Input: part model. Units: mm. Frame: model coordinates. A direction names the side the tool comes from. Give positions to 0.01 mm unless a question says otherwise; leave off trailing zeros. Order: outer loops, then holes, each group sorted by start corner. A loop starts at its lowest first (then second) coordinate and runs counter-clockwise, first axis right, second up.
```python
from build123d import *

# Parameters (mm, degrees)
F0_W           = 50
F0_H           = 45
F1_DEPTH       = 30
F2_SIZE        = 10
F4_D           = 8.8
F4_CBORE_D     = 14.25
F4_CBORE_DEPTH = 8
F5_DEPTH       = 50


with BuildPart() as f1:
    # F0 (on Top) → F1 (new body)
    with BuildSketch(Plane.XY):
        with Locations((-2.2690217942, 1.8614111841)):
            Rectangle(F0_W, F0_H)
    extrude(amount=F1_DEPTH)

    # F2
    f2_edges = [f1.edges().sort_by_distance(p)[0] for p in [
        (-27.269022, 24.361411, 15),
        (22.730978, -20.638589, 15),
        (22.730978, 24.361411, 15),
        (-27.269022, -20.638589, 15),
    ]]
    chamfer(f2_edges, length=F2_SIZE)

    # F4 (through all)
    with Locations(Plane.XY.offset(30)):
        with Locations((-17.6340711126, -7.961328021), (10.0047006537, 14.9650736012)):
            CounterBoreHole(F4_D / 2, F4_CBORE_D / 2, F4_CBORE_DEPTH)

    # F5 (add): a face of the model
    f5_faces = [f1.faces().sort_by_distance(p)[0] for p in [
        (-1.9842087331, 1.5591300529, 30),
    ]]
    extrude(f5_faces, amount=F5_DEPTH)


solid = f1.part
```
1) Cut plane A-A (x = 8.5). Return the cut outline in (y, z).
2) Line query: probe 1 along Y at (x, z) = (12.5, 50); probe 2 along X at (y, z) = (13.5, 31.5); probe 3 along X at (y, z) = (-9, 11). Output: solid intervals per line, ascending.
3) Cut plane D-D (z = 62). Return the cut outline in (x, y) (3 decimals).
4) Pull-direction query (X, two-part tool) for faces 1 (the face through (-3, 2, 80)), 2 (the face through (22.731, 2, 39)), 3 (the face through (10, 10, 22)); classes: pulls with the +X half, pulls with the -X half, needs draft (parallel to the pull), parting line crosses it, or undercut.
5) Cut plane C-C (y = -11.5). Return the cut outline in (x, z), then the cut area to 3 significant figures.
6) Reachability of faces 4 (the face through (-13, -8, 22)), 5 (the face through (-27.269, 2, 39)) from +Z, -Z, +X, -X, +Y, -Y: full face, straight path, thin tool, end or side. Return the list, or none.
7) Cut plane B-B (z = 17.5). Return the cut outline in (x, y).
8) First-contact query: P1, Ø4.5, axis at x = 8, y = 17, coming from the +Z side. Flat tip, straight axial feed; report the tip coordinate or a pass-through.
Geometry says:
1. outline: (-20.64, 0) - (10.83, 0) - (10.83, 22) - (8, 22) - (8, 80) - (-20.64, 80) - close; (19.1, 0) - (24.36, 0) - (24.36, 80) - (21.93, 80) - (21.93, 22) - (19.1, 22) - close
2. probe 1: y = -20.64 to 8.29, 21.64 to 24.36
2. probe 2: x = -27.27 to 3.03, 16.98 to 22.73
2. probe 3: x = -27.27 to -21.91, -13.36 to 22.73
3. outline: (-27.269, -10.639) - (-17.269, -20.639) - (12.731, -20.639) - (22.731, -10.639) - (22.731, 14.361) - (12.731, 24.361) - (-17.269, 24.361) - (-27.269, 14.361) - close; hole circle Ø14.25 at (-17.634, -7.961); hole circle Ø14.25 at (10.005, 14.965)
4. face 1: needs draft
4. face 2: pulls with the +X half
4. face 3: undercut
5. outline: (-26.41, 0) - (-20.25, 0) - (-20.25, 22) - (-23.82, 22) - (-23.82, 80) - (-26.41, 80) - close; (-15.02, 0) - (21.87, 0) - (21.87, 80) - (-11.45, 80) - (-11.45, 22) - (-15.02, 22) - close
5. area: 3,030 mm2
6. face 4: +Z
6. face 5: +Z, -Z, -X, +Y, -Y
7. outline: (-27.27, -10.64) - (-17.27, -20.64) - (12.73, -20.64) - (22.73, -10.64) - (22.73, 14.36) - (12.73, 24.36) - (-17.27, 24.36) - (-27.27, 14.36) - close; hole circle Ø8.8 at (-17.63, -7.96); hole circle Ø8.8 at (10, 14.97)
8. P1: stops at z = 22
